Geometry: final body of the model. Coordinates: model frame, mm. Face numbers are marked on the shaded views. Coordinates: 2 decimals unless noted, no trailing zeros. Loops run counter-clockwise (first coordinate to the right, second up) from the corner with the lowest first, then second, coordinate; pieces in that order, holes last. Notation, with made-up numbers: (78, 36) - (88, 36) arc R5 ccw to (88, 45) - close; hole circle Ø5 at (-36, 20). An arc over 180 degrees is marked (long way). Put each result on its own line as item: value. Start each with the question number.
1) Draft query along X for the marked faces 1, 2 and 3. Return one class per face: +X half, -X half, draft (parallel to the pull), parting line (faces both ways), or undercut.
2) Contact query for flat-ended pins moving along their axis: pin 1 Ø3.5 at (x, z) = (0, 19.5) entering from +Y; pin 2 Ø6 at (y, z) = (5, 2) entering from -X; pin 3 Ø6 at (y, z) = (3, -6) entering from -X; pin 4 Ø4 at (x, z) = (0, 0) entering from -Y. Output: stop coordinate, or through.
3) Material intervals for line 1 along X through (y, z) = (11.05, 0); line 2 along X through (y, z) = (9, -3); line 3 along Z through (x, y) = (0.5, 4.75), sorted ascending. Write a range as from..to.
4) Section A-A on y = 10.75. Output: boundary loops of the cut face in (x, z), and give its area (3 significant figures).
5) Section C-C on y = 1.25. Output: boundary loops of the cut face in (x, z).
6) Section B-B on z = 0. Output: boundary loops of the cut face in (x, y), and give its area (3 significant figures).
```python
from build123d import *

# Parameters (mm, degrees)
ESQUISSE1_R             = 31
ESQUISSE1_R_2           = 2.5
EXTRUSION1_DEPTH        = 13
ESQUISSE2_R             = 29.5
ESQUISSE2_R_2           = 9
ENL_V_MAT_EXTRU_1_DEPTH = 5
CONG_1_R                = 0.5
ESQUISSE3_R             = 1.5
ENL_V_MAT_EXTRU_2_DEPTH = 5


with BuildPart() as part:
    # Esquisse1 → Extrusion1 (new body)
    with BuildSketch(Plane(origin=(0, 0, 0), x_dir=(1, 0, 0), z_dir=(0, 1, 0))):
        with Locations(Location((0, 0, 0), (0, 0, 90))):
            Circle(ESQUISSE1_R)
        with Locations(Location((0, 0, 0), (0, 0, 90))):
            Circle(ESQUISSE1_R_2, mode=Mode.SUBTRACT)
    extrude(amount=EXTRUSION1_DEPTH)

    # Esquisse2 → Enlèv. mat.-Extru.1 (cut)
    with BuildSketch(Plane(origin=(0, 13, 0), x_dir=(1, 0, 0), z_dir=(0, 1, 0))):
        with Locations(Location((0, 0, 0), (0, 0, 270))):
            Circle(ESQUISSE2_R)
        with Locations(Location((0, 0, 0), (0, 0, 270))):
            Circle(ESQUISSE2_R_2, mode=Mode.SUBTRACT)
    extrude(amount=-ENL_V_MAT_EXTRU_1_DEPTH, mode=Mode.SUBTRACT)

    # Congé1
    cong_1_edges = [part.edges().sort_by_distance(p)[0] for p in [
        (0, 8, -29.5),
        (0, 8, -9),
        (0, 13, -29.5),
        (0, 13, -9),
        (0, 13, 31),
    ]]
    fillet(cong_1_edges, radius=CONG_1_R)

    # Esquisse3 → Enlèv. mat.-Extru.2 (cut)
    with BuildSketch(Plane(origin=(0, 8, 0), x_dir=(1, 0, 0), z_dir=(0, 1, 0))):
        with Locations(Location((0, 20, 0), (0, 0, 270))):
            Circle(ESQUISSE3_R)
        with Locations(Location((0, -20, 0), (0, 0, 270))):
            Circle(ESQUISSE3_R)
    extrude(amount=-ENL_V_MAT_EXTRU_2_DEPTH, mode=Mode.SUBTRACT)


solid = part.part
```
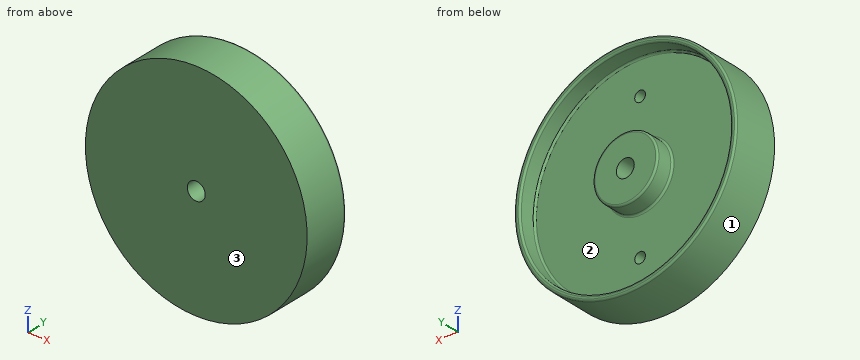
Answer block:
1. face 1: parting line
1. face 2: undercut
1. face 3: draft
2. pin 1: stops at y = 8
2. pin 2: stops at x = -31
2. pin 3: stops at x = -30.85
2. pin 4: passes through
3. line 1: x = -31..-29.5, -9..-2.5, 2.5..9, 29.5..31
3. line 2: x = -30.85..-29.35, -8.49..8.49, 29.35..30.85
3. line 3: z = -31..-21.41, -18.59..-2.45, 2.45..18.59, 21.41..31
4. outline: circle Ø62 at (0, 0); circle Ø18 at (0, 0); hole circle Ø59 at (0, 0); hole circle Ø5 at (0, 0)
4. area: 520 mm²
5. outline: circle Ø62 at (0, 0); hole circle Ø5 at (0, 0)
6. outline: (-31, 0) - (-2.5, 0) - (-2.5, 13) - (-8.5, 13) arc R0.5 ccw to (-9, 12.5) - (-9, 8.5) arc R0.5 cw to (-9.5, 8) - (-29, 8) arc R0.5 cw to (-29.5, 8.5) - (-29.5, 12.5) arc R0.5 ccw to (-30, 13) - (-30.5, 13) arc R0.5 ccw to (-31, 12.5) - close; (2.5, 0) - (31, 0) - (31, 12.5) arc R0.5 ccw to (30.5, 13) - (30, 13) arc R0.5 ccw to (29.5, 12.5) - (29.5, 8.5) arc R0.5 cw to (29, 8) - (9.5, 8) arc R0.5 cw to (9, 8.5) - (9, 12.5) arc R0.5 ccw to (8.5, 13) - (2.5, 13) - close
6. area: 536 mm²
